from build123d import *

# Parameters (mm, degrees)
IZIM1_R                     = 5
Y_KSEKLIK_EKSTR_ZYON2_DEPTH = 1
IZIM2_R                     = 3
Y_KSEKLIK_EKSTR_ZYON4_DEPTH = 1


with BuildPart() as part:
    # Çizim1 → Yükseklik-Ekstrüzyon2 (new body)
    with BuildSketch(Plane.XY):
        with BuildLine():
            Line((-16.200531831, -56.860261047), (-16.200531831, 33.139738953))
            Line((-16.200531831, 33.139738953), (-25, 33.139738953))
            Line((-25, 33.139738953), (-25, -57.883306535))
            ThreePointArc((-25, -57.883306535), (-18.410044855, -76.210418758), (-16.200531831, -56.860261047))
        make_face()
        with Locations((-19.564888058, -66.277325727)):
            Circle(IZIM1_R, mode=Mode.SUBTRACT)
    extrude(amount=Y_KSEKLIK_EKSTR_ZYON2_DEPTH)

    # Çizim2 → Yükseklik-Ekstrüzyon4 (add)
    with BuildSketch(Plane.XY.offset(1)):
        with BuildLine():
            Line((-14.268162917, -55.859645389), (-13.746523784, -58.818007922))
            ThreePointArc((-13.746523784, -58.818007922), (-13.437306239, -59.381637082), (-12.848871774, -59.640554443))
            Line((-12.848871774, -59.640554443), (-9.856302857, -59.902370298))
            ThreePointArc((-9.856302857, -59.902370298), (-8.217998769, -61.049523171), (-8.392310254, -63.041912567))
            Line((-8.392310254, -63.041912567), (-10.115333894, -65.502645344))
            ThreePointArc((-10.115333894, -65.502645344), (-10.295230071, -66.119841167), (-10.062226293, -66.71900939))
            Line((-10.062226293, -66.71900939), (-8.131292285, -69.02020693))
            ThreePointArc((-8.131292285, -69.02020693), (-7.78399593, -70.989822436), (-9.316084816, -72.275397656))
            Line((-9.316084816, -72.275397656), (-12.274447349, -72.797036789))
            ThreePointArc((-12.274447349, -72.797036789), (-12.838076508, -73.106254334), (-13.09699387, -73.694688799))
            Line((-13.09699387, -73.694688799), (-13.358809725, -76.687257716))
            ThreePointArc((-13.358809725, -76.687257716), (-14.505962597, -78.325561805), (-16.498351994, -78.151250319))
            Line((-16.498351994, -78.151250319), (-18.95908477, -76.428226679))
            ThreePointArc((-18.95908477, -76.428226679), (-19.576280594, -76.248330502), (-20.175448817, -76.48133428))
            Line((-20.175448817, -76.48133428), (-22.476646357, -78.412268288))
            ThreePointArc((-22.476646357, -78.412268288), (-24.446261863, -78.759564643), (-25.731837083, -77.227475757))
            Line((-25.731837083, -77.227475757), (-26.253476216, -74.269113224))
            ThreePointArc((-26.253476216, -74.269113224), (-26.562693761, -73.705484065), (-27.151128226, -73.446566704))
            Line((-27.151128226, -73.446566704), (-30.143697143, -73.184750849))
            ThreePointArc((-30.143697143, -73.184750849), (-31.782001231, -72.037597976), (-31.607689746, -70.04520858))
            Line((-31.607689746, -70.04520858), (-29.884666106, -67.584475803))
            ThreePointArc((-29.884666106, -67.584475803), (-29.704769929, -66.967279979), (-29.937773707, -66.368111757))
            Line((-29.937773707, -66.368111757), (-31.868707715, -64.066914216))
            ThreePointArc((-31.868707715, -64.066914216), (-32.21600407, -62.09729871), (-30.683915184, -60.811723491))
            Line((-30.683915184, -60.811723491), (-27.725552651, -60.290084357))
            ThreePointArc((-27.725552651, -60.290084357), (-27.161923492, -59.980866812), (-26.90300613, -59.392432347))
            Line((-26.90300613, -59.392432347), (-26.641190275, -56.39986343))
            ThreePointArc((-26.641190275, -56.39986343), (-25.494037403, -54.761559342), (-23.501648006, -54.935870827))
            Line((-23.501648006, -54.935870827), (-21.04091523, -56.658894467))
            ThreePointArc((-21.04091523, -56.658894467), (-20.423719406, -56.838790644), (-19.824551183, -56.605786866))
            Line((-19.824551183, -56.605786866), (-17.523353643, -54.674852858))
            ThreePointArc((-17.523353643, -54.674852858), (-15.553738137, -54.327556503), (-14.268162917, -55.859645389))
        make_face()
        with Locations((-20, -66.543560573)):
            Circle(IZIM2_R, mode=Mode.SUBTRACT)
    extrude(amount=-Y_KSEKLIK_EKSTR_ZYON4_DEPTH)


solid = part.part
Read the model definition and answer for the solid it produces. Units are mm, in the model's axes. A direction names the side the tool comes from. Give positions to 0.01 mm unless a question says otherwise; leave off trailing zeros. Write each loop counter-clockwise with the first axis right and the second up, starting at its lowest first coordinate (ties: lowest second). Pieces come first, ordered by that corner, then holes. Notation, with made-up numbers: (56.5, 56.25) - (93.5, 56.25) arc R18 cw to (93.5, 86.25) - close; hole circle Ø3 at (7.25, -15). An arc over 180 degrees is marked (long way). Answer in a Markdown table with one row per item. Add a question column.
Item 1: Section B-B, the plane x = -11 is taken. Write down the section's boundary in (y, z).
Item 2: Find the intervals of material crossed by L1, parallel to X at y = 2, z = 0.15; L2, parallel to Y at x = -20, z = 0.45; L3, parallel to Y at x = -11.25, z = 0.1, in increasing order.
Item 3: Section A-A, the plane y = -29 is taken. Write down the section's boundary in (x, z).
Item 4: Flat-ended cylindrical pins translate along their axes: P1, Ø6, axis at x = -28.5, y = -48, coming from the +Z side; P2, Ø0.5, axis at y = -21, z = 0.5, coming from the -X side. Find the tip coordinate at first contact, or state that the pin passes through.
Item 5: Determine the mould class of faces 4 (the face through (-14.479, -78.313, 0.507)), 5 (the face through (-20, -35, 1)), 6 (the face through (-30.758, -68.832, 0.507)) for opening direction Y: pulls with the +Y half, pulls with the -Y half, needs draft (parallel to the pull), parting line crosses it, or undercut.
Item 6: A tool of negligible diameter and unlimited length cuts with its end or side. For faces 1 (the face through (-21.31, -77.433, 0.507)), 2 (the face through (-30.89, -65.234, 0.507)), 3 (the face through (-8.23, -61.02, 0.51)), from which of +Z, -Z, +X, -X, +Y, -Y can it reach the whole face along a straight path? Write none if from no direction.
Recorded:
| question | item | result |
|---|---|---|
| 1 | outline | (-72.57, 0) - (-59.8, 0) - (-59.8, 1) - (-72.57, 1) - close |
| 2 | L1 | x = -25 to -16.2 |
| 2 | L2 | y = -76.36 to -69.54, -63.54 to 33.14 |
| 2 | L3 | y = -72.62 to -59.78 |
| 3 | outline | (-25, 0) - (-16.2, 0) - (-16.2, 1) - (-25, 1) - close |
| 4 | P1 | passes through |
| 4 | P2 | stops at x = -25 |
| 5 | face 4 | pulls with the -Y half |
| 5 | face 5 | needs draft |
| 5 | face 6 | undercut |
| 6 | face 1 | +Z, -Z, -Y |
| 6 | face 2 | +Z, -Z, -X |
| 6 | face 3 | +Z, -Z, +X |
